The listing builds one solid part. Answer for the finished solid, in the listing's coordinates (mm). A direction names the side the tool comes from. Round coordinates to 2 decimals unless told otherwise and drop trailing zeros. Order: outer loops, then holes, each group sorted by start corner. A loop starts at its lowest first (then second) coordinate and runs counter-clockwise, first axis right, second up. Notation, with made-up numbers: (71, 5.25) - (109, 5.25) arc R14 cw to (109, 11.25) - close; hole circle Ø4 at (-8.75, 64). An arc over 180 degrees is marked (long way). Write item = value, one per line.
Autodesk Inventor part; units mm, degrees
ref_plane "YZ Plane" through (0, 0, 0) normal (1, 0, 0) x (0, 1, 0)
ref_plane "XZ Plane" through (0, 0, 0) normal (0, 1, 0) x (-1, 0, 0)
ref_plane "XY Plane" through (0, 0, 0) normal (0, 0, 1) x (1, 0, 0)
sketch "スケッチ1" plane through (0, 0, 0) normal (0, 0, 1) x (1, 0, 0)
  line L0 (26.25, -10.5) -> (-26.25, -10.5)
  line L1 (-26.25, -10.5) -> (-26.25, 10.5)
  line L2 (-26.25, 10.5) -> (26.25, 10.5)
  line L3 (26.25, 10.5) -> (26.25, -10.5)
  line L4 (26.25, -10.5) -> (-26.25, 10.5) construction
  line L5 (-26.25, -10.5) -> (26.25, 10.5) construction
  point P0 (0, 0)
  dimension "d0" = 52.5
  dimension "d2" = 21
extrude "押し出し1" add sketch "スケッチ1" along normal blind 8.5
sketch "スケッチ19" plane through (0, 0, 0) normal (0, 0, -1) x (-1, 0, 0)
  circle A0 centre (-22.25, 5.5) radius 1.1
  circle A1 centre (22.25, 5.5) radius 1.1
  circle A2 centre (22.25, -5.5) radius 1.1
  circle A3 centre (-22.25, -5.5) radius 1.1
  point P0 (0, 0)
  dimension "d140" = 2.2
  dimension "d141" = 2.2
  dimension "d142" = 2.2
  dimension "d143" = 2.2
  dimension "d144" = 44.5
  dimension "d145" = 22.25
  dimension "d146" = 11
  dimension "d147" = 5.5
  dimension "d148" = 44.5
  dimension "d149" = 11
extrude "押し出し15" cut sketch "スケッチ19" against normal through all
sketch "スケッチ20" plane through (0, 0, 8.5) normal (0, 0, 1) x (1, 0, 0)
  line L0 (25, -8.75) -> (-25, -8.75)
  line L1 (-25, -8.75) -> (-25, 8.75)
  line L2 (-25, 8.75) -> (25, 8.75)
  line L3 (25, 8.75) -> (25, -8.75)
  point P0 (0, 0)
  dimension "d152" = 50
  dimension "d153" = 25
  dimension "d154" = 17.5
  dimension "d155" = 8.75
extrude "押し出し16" cut sketch "スケッチ20" against normal blind 6.5
sketch "スケッチ21" plane through (26.25, -10.5, 0) normal (1, 0, 0) x (0, 0, -1)
  line L0 (-8.5, 0) -> (-8.5, 21)
  line L1 (-8.5, 14.5) -> (-4, 14.5)
  line L2 (-4, 14.5) -> (-4, 6.5)
  line L3 (-4, 6.5) -> (-8.5, 6.5)
  line L4 (-8.5, 6.5) -> (-8.5, 14.5)
  line L5 (0, 21) -> (-8.5, 21)
  line L6 (0, 0) -> (-8.5, 0)
  line L7 (0, 21) -> (0, 0)
  point P0 (0, 10.5)
  dimension "d160" = 4
  dimension "d163" = 6.5
  dimension "d164" = 6.5
extrude "押し出し17" cut sketch "スケッチ21" against normal blind 7 contours L0 L1 L2 L3
sketch "スケッチ22" plane through (0, 0, 0) normal (0, 0, -1) x (-1, 0, 0)
  circle A0 centre (10.5, 0) radius 9.5
  circle A1 centre (-10.5, 0) radius 9.5
  point P0 (0, 0)
  dimension "d165" = 19
  dimension "d166" = 19
  dimension "d167" = 10.5
  dimension "d168" = 10.5
extrude "押し出し18" cut sketch "スケッチ22" against normal through all
fillet "フィレット3" radius 1 8 edges at (-26.25, 10.5, 4.25) (-26.25, 0, 0) (-26.25, -10.5, 4.25) (0, 10.5, 0) (26.25, 10.5, 4.25) (26.25, 0, 0) (0, -10.5, 0) (26.25, -10.5, 4.25)
properties part number "New_Accelite_Controller_Cover_copy" material "ABS プラスチック"
Q1. Section C-C on z = 0.5 is taken. Determine the outline of the cut face in (x, y), then the cut area to 3 significant figures.
Model answer:
outline = (-26.12, -9.5) arc R0.87 ccw to (-25.25, -10.37) - (25.25, -10.37) arc R0.87 ccw to (26.12, -9.5) - (26.12, 9.5) arc R0.87 ccw to (25.25, 10.37) - (-25.25, 10.37) arc R0.87 ccw to (-26.12, 9.5) - close; hole circle Ø2.2 at (-22.25, -5.5); hole circle Ø2.2 at (-22.25, 5.5); hole circle Ø19 at (-10.5, 0); hole circle Ø19 at (10.5, 0); hole circle Ø2.2 at (22.25, -5.5); hole circle Ø2.2 at (22.25, 5.5)
area = 500 mm^2
Q2. Section B-B on y = 8.25 is taken. Determine the outline of the cut face in (x, z).
Model answer:
outline = (-26.25, 1) arc R1 ccw to (-25.25, 0) - (-15.21, 0) - (-15.21, 2) - (-25, 2) - (-25, 8.5) - (-26.25, 8.5) - close; (-5.79, 0) - (5.79, 0) - (5.79, 2) - (-5.79, 2) - close; (15.21, 0) - (25.25, 0) arc R1 ccw to (26.25, 1) - (26.25, 8.5) - (25, 8.5) - (25, 2) - (15.21, 2) - close
Q3. For faces 1 (the face through (-21.15, 5.55, 0.99)), 2 (the face through (26, -4, 6)), 3 (the face through (0, 0, 2)), determine the directions among +Z, -Z, +X, -X, +Y, -Y from which every point of the face is accessible in a straight line to the end or side of a thin tool.
Model answer:
face_1 = +Z, -Z
face_2 = +Z, +X
face_3 = +Z
Q4. Flat-ended cylindrical pins translate along their axes: P1, Ø3, axis at x = -22.25, y = -5.5, coming from the +Z side; P2, Ø2, axis at y = 1.5, z = 6.5, coming from the +X side. Find the tip coordinate at first contact, or state that the pin passes through.
Model answer:
P1 = 2
P2 = -25
Q5. Determine the mould class of faces 4 (the face through (25, 0, 3)), 5 (the face through (0, -10.5, 5)), 6 (the face through (25.965, 10.199, 4.802)) for opening direction Y: released by +Y, released by -Y, zero draft, split by the parting line, or undercut.
Model answer:
face_4 = undercut
face_5 = released by -Y
face_6 = released by +Y
Q6. Find the intervals of material crossed by line 1 (Y direction, x = -22.25, z = 0.95); line 2 (X direction, y = 2.5, z = 3); line 3 (Y direction, x = 10.5, z = 2.5), in increasing order. Write a range as from..to.
Model answer:
line_1 = -10.5..-6.6, -4.4..4.4, 6.6..10.5
line_2 = -26.25..-25, 25..26.25
line_3 = -10.5..-9.5, 9.5..10.5
Q7. Section A-A on x = -22.25 is taken. Determine the outline of the cut face in (y, z), then the cut area to 3 significant figures.
Model answer:
outline = (-10.5, 1) arc R1 ccw to (-9.5, 0) - (-6.6, 0) - (-6.6, 2) - (-8.75, 2) - (-8.75, 8.5) - (-10.5, 8.5) - close; (-4.4, 0) - (4.4, 0) - (4.4, 2) - (-4.4, 2) - close; (6.6, 0) - (9.5, 0) arc R1 ccw to (10.5, 1) - (10.5, 8.5) - (8.75, 8.5) - (8.75, 2) - (6.6, 2) - close
area = 55.5 mm^2
